```python
from build123d import *

# Parameters (mm, degrees)
EXTRUDE_THIN1_DEPTH  = 30
M8_CLEARANCE_HOLE1_D = 10
CUT_EXTRUDE1_REACH   = 72.491
FILLET1_R            = 1


with BuildPart() as part:
    # Sketch1 → Extrude-Thin1 (new, symmetric)
    with BuildSketch(Plane.XY):
        Polygon((0, 0), (30, 0), (30, 12), (35, 12), (35, -5), (0, -5), align=None)
    extrude(amount=EXTRUDE_THIN1_DEPTH, both=True)

    # M8 Clearance Hole1 (through all)
    with Locations(Plane(origin=(0, -5, 0), x_dir=(-1, 0, 0), z_dir=(0, -1, 0))):
        with Locations((-15, 15), (-15, -15)):
            Hole(M8_CLEARANCE_HOLE1_D / 2)

    # Sketch5 → Cut-Extrude1 (cut, up to next)
    with BuildSketch(Plane(origin=(0, 0, -30), x_dir=(-1, 0, 0), z_dir=(0, 0, -1)), mode=Mode.PRIVATE) as cut_extrude1_sk1:
        Polygon((-30, 0), (-31, 0), (-31, 1), (-30, 2), align=None)
    cut_extrude1_tool1 = extrude(cut_extrude1_sk1.sketch, amount=-CUT_EXTRUDE1_REACH, mode=Mode.PRIVATE) & part.part
    add(cut_extrude1_tool1.solids().sort_by_distance((30.444444, 0.777778, -30))[0], mode=Mode.SUBTRACT)

    # Fillet1
    fillet1_edges = [part.edges().sort_by_distance(p)[0] for p in [
        (0, -2.5, 30),
        (35, 3.5, 30),
        (0, -2.5, -30),
        (32.5, 12, -30),
        (35, 3.5, -30),
        (32.5, 12, 30),
    ]]
    fillet(fillet1_edges, radius=FILLET1_R)


solid = part.part
```
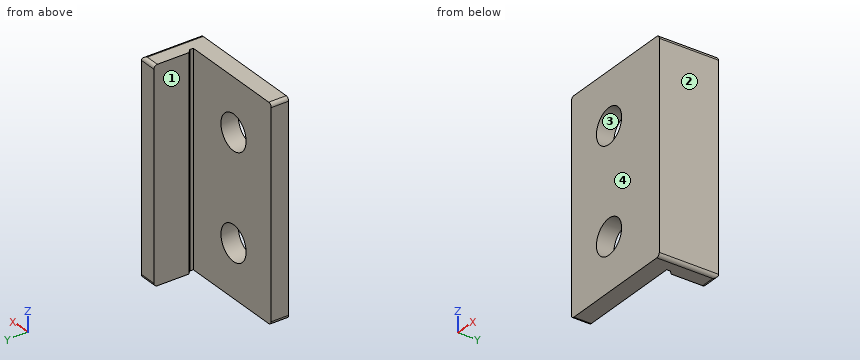
Source: CAD feature listing. Evaluate the final solid. Frame: model axes, mm. Face numbers are marked on the shaded views. A direction names the side the tool comes from. Coordinates: 2 decimals unless noted, no trailing zeros. Write each loop counter-clockwise with the first axis right and the second up, starting at its lowest first coordinate (ties: lowest second). Pieces come first, ordered by that corner, then holes. Notation, with made-up numbers: M 16,-25.75 L 46,-25.75 A17 ccw 46,-17.75 Z; hole C -27,-33.5 d5. An arc over 180 degrees is marked long. Answer as a JSON object with one key per item and string values.
1. Cut plane B-B on x = 15. Output: boundary loops of the cut face in (y, z), plus the area to 3 significant figures.
Evaluation:
{"outline": "M -5,-30 L 0,-30 L 0,-20 L -5,-20 Z; M -5,-10 L 0,-10 L 0,10 L -5,10 Z; M -5,20 L 0,20 L 0,30 L -5,30 Z", "area": "200 mm^2"}
2. Access query for the marked faces 1 and 2. Directions: +Z, -Z, +X, -X, +Y, -Y. A direction counts if a zero-diameter tool reaches every point of the face in a straight line with its end or side. Return the directions, or none.
Evaluation:
{"face 1": "+Z, -Z, -X, +Y", "face 2": "+Z, -Z, +X, +Y, -Y"}
3. Cut plane C-C on z = -15. Output: boundary loops of the cut face in (x, y), plus the area to 4 significant figures.
Evaluation:
{"outline": "M 0,-5 L 10,-5 L 10,0 L 0,0 Z; M 20,-5 L 35,-5 L 35,12 L 30,12 L 30,2 L 31,1 L 31,0 L 20,0 Z", "area": "183.5 mm^2"}
4. Contact query for flat-ended pins moving along their axis: P1, Ø0.8, axis at y = 0.5, z = -1.5, coming from the -X side; P2, Ø13, axis at x = 15, z = 15, coming from the +Y side; P3, Ø8, axis at x = 15, z = -15, coming from the -Y side; P4, Ø5, axis at y = 8, z = -3.5, coming from the -X side. Output: stop coordinate, or through.
Evaluation:
{"P1": "x = 31", "P2": "y = 0", "P3": "through", "P4": "x = 30"}
5. Draft query along Z for the marked faces 3 and 4. Return one class per face: released by +Z, released by -Z, zero draft, split by the parting line, or undercut.
Evaluation:
{"face 3": "undercut", "face 4": "zero draft"}
6. Cut plane D-D on z = -5. Output: boundary loops of the cut face in (x, y).
Evaluation:
{"outline": "M 0,-5 L 35,-5 L 35,12 L 30,12 L 30,2 L 31,1 L 31,0 L 0,0 Z"}
7. Ray query, L1, parallel to Z at x = 15, y = -1.4; L2, parallel to Z at x = 11, y = -3.5; L3, parallel to Y at x = 19, z = -9.5. Return the intervals inside material, ascending.
Evaluation:
{"L1": "-30 to -20, -10 to 10, 20 to 30", "L2": "-30 to -18, -12 to 12, 18 to 30", "L3": "-5 to 0"}
8. Cut plane A-A on y = -1. Output: boundary loops of the cut face in (x, z).
Evaluation:
{"outline": "M 0,-29 A1 ccw 1,-30 L 34,-30 A1 ccw 35,-29 L 35,29 A1 ccw 34,30 L 1,30 A1 ccw 0,29 Z; hole C 15,-15 d10; hole C 15,15 d10"}
